```python
from build123d import *

# Parameters (mm, degrees)
SKETCH1_R           = 25
BOSS_EXTRUDE1_DEPTH = 10
BOSS_EXTRUDE3_DEPTH = 27.5
SKETCH7_W           = 40
SKETCH7_H           = 96.533506044
CUT_EXTRUDE3_DEPTH  = 55
CHAMFER1_SIZE       = 3
SKETCH8_R           = 17.5
BOSS_EXTRUDE4_DEPTH = 40
CHAMFER2_SIZE       = 5


with BuildPart() as part:
    # Sketch1 → Boss-Extrude1 (new body)
    with BuildSketch(Plane.XY):
        Circle(SKETCH1_R)
    extrude(amount=BOSS_EXTRUDE1_DEPTH)

    # Sketch6 → Boss-Extrude3 (add, symmetric)
    with BuildSketch(Plane(origin=(0, 0, 0), x_dir=(0, 0, -1), z_dir=(1, 0, 0))):
        with BuildLine():
            Line((10, 20), (60, 20))
            ThreePointArc((60, 20), (80, 0), (60, -20))
            Line((60, -20), (10, -20))
            ThreePointArc((10, -20), (-10, 0), (10, 20))
        make_face()
    extrude(amount=BOSS_EXTRUDE3_DEPTH, both=True)

    # Sketch7 → Cut-Extrude3 (cut)
    with BuildSketch(Plane(origin=(0, 20, 0), x_dir=(1, 0, 0), z_dir=(0, 1, 0))):
        with Locations((0, 48.266753022)):
            Rectangle(SKETCH7_W, SKETCH7_H)
    extrude(amount=-CUT_EXTRUDE3_DEPTH, mode=Mode.SUBTRACT)

    # Chamfer1
    # the kernel refuses this chamfer: 3 mm, written as the material it takes off along each edge
    with BuildSketch(Plane(origin=(-27.5, -20, -60), x_dir=(0.9996219169112965, -0.02749587661058676, 0), z_dir=(0, 0, 1)), Plane(origin=(27.5, -20, -60), x_dir=(0.027495876610586768, 0.9996219169112968, 0), z_dir=(0, 0, 1)), Plane(origin=(27.5, 20, -10), x_dir=(0.027495876610586768, -0.9996219169112968, 0), z_dir=(0, 0, -1))) as chamfer1_piece_1:
        Polygon((CHAMFER1_SIZE * 0.999621916911, CHAMFER1_SIZE * 0.0274958766106), (-CHAMFER1_SIZE * 0.0274958766106, CHAMFER1_SIZE * 0.999621916911), (0, 0), align=None)
    extrude(amount=50, mode=Mode.SUBTRACT)
    with BuildSketch(Plane(origin=(-27.5, 0, -60), x_dir=(0, 1, 0), z_dir=(0, 0, 1))) as chamfer1_piece_2:
        Polygon((20 - CHAMFER1_SIZE, 0), (20, -CHAMFER1_SIZE), (20, 0), align=None)
    revolve(axis=Axis((-27.5, 0, -60), (-1, 0, 0)), revolution_arc=180, mode=Mode.SUBTRACT)
    with BuildSketch(Plane(origin=(-27.5, 0, -10), x_dir=(0, -1, 0), z_dir=(0, 0, -1))) as chamfer1_piece_3_section:
        Polygon((20 - CHAMFER1_SIZE, 0), (20, -CHAMFER1_SIZE), (20, 0), align=None)
    chamfer1_piece_3 = revolve(axis=Axis((-27.5, 0, -10), (-1, 0, 0)), revolution_arc=180, mode=Mode.PRIVATE)
    chamfer1_piece_3 = chamfer1_piece_3 - Plane(origin=(0, 0, 8.545585815), x_dir=(1, 0, 0), z_dir=(0, 0, -1)) * Cylinder(25, 81, mode=Mode.PRIVATE)
    add(chamfer1_piece_3, mode=Mode.SUBTRACT)
    with BuildSketch(Plane(origin=(-27.5, 20, -10), x_dir=(-0.027495876610586768, -0.9996219169112968, 0), z_dir=(0, 0, -1))) as chamfer1_piece_4:
        Polygon((CHAMFER1_SIZE * 0.999621916911, -CHAMFER1_SIZE * 0.0274958766106), (-CHAMFER1_SIZE * 0.0274958766106, -CHAMFER1_SIZE * 0.999621916911), (0, 0), align=None)
    extrude(amount=50, mode=Mode.SUBTRACT)
    with BuildSketch(Plane(origin=(27.5, 0, -60), x_dir=(0, 1, 0), z_dir=(0, 0, 1))) as chamfer1_piece_5:
        Polygon((20, CHAMFER1_SIZE), (20 - CHAMFER1_SIZE, 0), (20, 0), align=None)
    revolve(axis=Axis((27.5, 0, -60), (-1, 0, 0)), revolution_arc=180, mode=Mode.SUBTRACT)
    with BuildSketch(Plane(origin=(27.5, 0, -10), x_dir=(0, -1, 0), z_dir=(0, 0, -1))) as chamfer1_piece_6_section:
        Polygon((20 - CHAMFER1_SIZE, 0), (20, CHAMFER1_SIZE), (20, 0), align=None)
    chamfer1_piece_6 = revolve(axis=Axis((27.5, 0, -10), (-1, 0, 0)), revolution_arc=180, mode=Mode.PRIVATE)
    chamfer1_piece_6 = chamfer1_piece_6 - Plane(origin=(0, 0, 8.545585813), x_dir=(1, 0, 0), z_dir=(0, 0, -1)) * Cylinder(25, 81, mode=Mode.PRIVATE)
    add(chamfer1_piece_6, mode=Mode.SUBTRACT)

    # Sketch8 → Boss-Extrude4 (add)
    with BuildSketch(Plane(origin=(-20, 0, 0), x_dir=(0, 0, -1), z_dir=(1, 0, 0))):
        with Locations(Location((60, 0, 0), (0, 0, 180))):
            Circle(SKETCH8_R)
    extrude(amount=BOSS_EXTRUDE4_DEPTH)

    # Chamfer2
    chamfer2_edges = [part.edges().sort_by_distance(p)[0] for p in [
        (0, 25, 0),
        (0, -25, 0),
    ]]
    chamfer(chamfer2_edges, length=CHAMFER2_SIZE)


solid = part.part
```
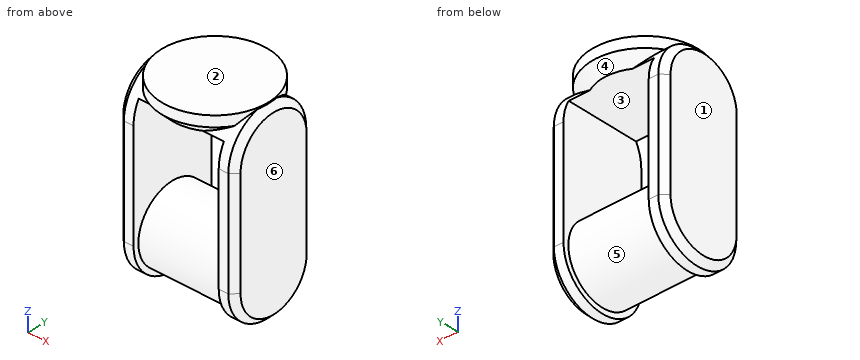
Source: CAD feature listing. Evaluate the final solid. Frame: model axes, mm. Face numbers are marked on the shaded views. A direction names the side the tool comes from. Coordinates: 2 decimals unless noted, no trailing zeros. Loops run counter-clockwise (first coordinate to the right, second up) from the corner with the lowest first, then second, coordinate; pieces in that order, holes last. Notation, with made-up numbers: M -4.5,23 L 29.5,23 A32 ccw 29.5,52 Z; hole C -33,-22 d11. An arc over 180 degrees is marked long. Use a Markdown table: item, result. Add a question column.
Q1. Section query C-C, the plane z = -55. Return loops of the section in (x, y), and give its area (3 significant figures).
Q2. Draft query along Z for the marked faces 1, 2 and 3. Return one class per face: pulls with the +Z half, pulls with the -Z half, needs draft (parallel to the pull), parting line crosses it, or undercut.
Q3. Material intervals for L1, parallel to X at y = 16.5, z = -38.5; L2, parallel to Z at x = -16, y = 9; L3, parallel to Z at x = 14.5, y = 11, sorted ascending.
Q4. First-contact query: pin 1 (10 mm diameter, centred on x = 13, y = -2, fed in from -Z); pin 2 (3.5 mm diameter, centred on x = -22.5, z = -45, fed in from -Y); pin 3 (1.5 mm diameter, centred on y = -19, z = -32.5, fed in from +X). Flat tips, straight axial feed; report the tip coordinate or a pass-through.
Q5. Section query A-A, the plane z = -14.5. Return loops of the section in (x, y), and give its area (3 significant figures).
Q6. Access query for the marked faces 4, 5 and 6. Directions: +Z, -Z, +X, -X, +Y, -Y. A direction counts if a zero-diameter tool reaches every point of the face in a straight line with its end or side. Return the directions, or none.
Q7. Section query B-B, the plane x = 0. Return loops of the section in (y, z).
Result:
| question | item | result |
|---|---|---|
| 1 | outline | M -27.5,-17 L -24.5,-20 L -20,-20 L -20,-16.77 L 20,-16.77 L 20,-20 L 24.5,-20 L 27.5,-17 L 27.5,17 L 24.5,20 L 20,20 L 20,16.77 L -20,16.77 L -20,20 L -24.5,20 L -27.5,17 Z |
| 1 | area | 1,920 mm2 |
| 2 | face 1 | needs draft |
| 2 | face 2 | pulls with the +Z half |
| 2 | face 3 | undercut |
| 3 | L1 | x = -27.5 to -20, 20 to 27.5 |
| 3 | L2 | z = -75.01 to -44.99, 0 to 10 |
| 3 | L3 | z = -73.61 to -46.39, 0 to 10 |
| 4 | pin 1 | stops at z = -77.5 |
| 4 | pin 2 | stops at y = -20 |
| 4 | pin 3 | stops at x = 26.25 |
| 5 | outline | M -27.5,-17 L -24.5,-20 L -20,-20 L -20,20 L -24.5,20 L -27.5,17 Z; M 20,-20 L 24.5,-20 L 27.5,-17 L 27.5,17 L 24.5,20 L 20,20 Z |
| 5 | area | 582 mm2 |
| 6 | face 4 | +Y |
| 6 | face 5 | none |
| 6 | face 6 | +Z, -Z, +X, +Y, -Y |
| 7 | outline | M -25,5 L -20,0 L 20,0 L 25,5 L 25,10 L -25,10 Z; C 0,-60 d35 |
